Source: CAD feature listing. Evaluate the final solid. Frame: model axes, mm. A direction names the side the tool comes from. Give positions to 0.01 mm unless a question says otherwise; leave off trailing zeros. Order: outer loops, then holes, each group sorted by start corner. A loop starts at its lowest first (then second) coordinate and runs counter-clockwise, first axis right, second up.
```python
from build123d import *

# Parameters (mm, degrees)
SKETCH001_W   = 180
SKETCH001_H   = 136
SKETCH001_W_2 = 164.9
SKETCH001_H_2 = 124.27
PAD001_DEPTH  = 10
SKETCH_W      = 170
SKETCH_H      = 127
SKETCH_W_2    = 165
SKETCH_H_2    = 100
PAD_DEPTH     = 10
SKETCH002_R   = 1.5
POCKET_DEPTH  = 7
CHAMFER_SIZE  = 1


with BuildPart() as body001:
    # Sketch001 → Pad001 (new body)
    with BuildSketch(Plane.XY):
        Rectangle(SKETCH001_W, SKETCH001_H)
        Rectangle(SKETCH001_W_2, SKETCH001_H_2, mode=Mode.SUBTRACT)
    extrude(amount=PAD001_DEPTH)


with BuildPart() as body001_1:
    # Body001 placement: moved
    add(body001.part.moved(Location((0, 0, 2))))


with BuildPart() as bezel:
    # Sketch → Pad (new body)
    with BuildSketch(Plane.XY):
        Rectangle(SKETCH_W, SKETCH_H)
        Rectangle(SKETCH_W_2, SKETCH_H_2, mode=Mode.SUBTRACT)
    extrude(amount=PAD_DEPTH)

    # Boolean: cut Body001
    add(body001_1.part, mode=Mode.SUBTRACT)

    # Sketch002 (on Face18 of Boolean) → Pocket (cut)
    with BuildSketch(Plane.XY.offset(10)):
        with Locations((-78.09, 56.795)):
            Circle(SKETCH002_R)
        with Locations((78.09, 56.795)):
            Circle(SKETCH002_R)
        with Locations((78.09, -56.795)):
            Circle(SKETCH002_R)
        with Locations((-78.09, -56.795)):
            Circle(SKETCH002_R)
    extrude(amount=-POCKET_DEPTH, mode=Mode.SUBTRACT)

    # Chamfer
    chamfer_edges = [bezel.edges().sort_by_distance(p)[0] for p in [
        (82.5, 0, 0),
        (0, -50, 0),
        (0, -63.5, 0),
        (85, 0, 0),
        (0, 63.5, 0),
        (-85, 0, 0),
        (0, 50, 0),
        (-82.5, 0, 0),
    ]]
    chamfer(chamfer_edges, length=CHAMFER_SIZE)


solid = bezel.part
```
1) Section query C-C, the plane x = -18. Return the cut outline in (y, z) (3 decimals).
Report:
outline: (-63.5, 1) - (-62.5, 0) - (-51, 0) - (-50, 1) - (-50, 10) - (-62.135, 10) - (-62.135, 2) - (-63.5, 2) - close; (50, 1) - (51, 0) - (62.5, 0) - (63.5, 1) - (63.5, 2) - (62.135, 2) - (62.135, 10) - (50, 10) - close
2) Draft query along Y for faces 5 (the flat face through (-1, 62.135, 6)), 6 (the flat face through (-82.45, 56, 6)), 7 (the flat face through (-1, -50, 5)). Return one class per face: +Y half, -Y half, draft (parallel to the pull), parting line (faces both ways), or undercut.
Report:
face 5: +Y half
face 6: draft
face 7: undercut
3) Section query B-B, the plane z = 8.25. Return the cut outline in (x, y) (3 decimals), and give its area (3 significant figures).
Report:
outline: (-82.45, -62.135) - (82.45, -62.135) - (82.45, -50) - (-82.45, -50) - close; (-82.45, 50) - (82.45, 50) - (82.45, 62.135) - (-82.45, 62.135) - close; hole circle Ø3 at (-78.09, -56.795); hole circle Ø3 at (-78.09, 56.795); hole circle Ø3 at (78.09, -56.795); hole circle Ø3 at (78.09, 56.795)
area: 3,970 mm2
4) Material intervals for L1, parallel to Y at x = 78.09, z = 4.75 (3 decimals); L2, parallel to Y at x = 63, z = 5.5 (3 decimals); L3, parallel to X at y = 53.5, z = 6.5, sorted ascending.
Report:
L1: y = -62.135 to -58.295, -55.295 to -50, 50 to 55.295, 58.295 to 62.135
L2: y = -62.135 to -50, 50 to 62.135
L3: x = -82.45 to 82.45
5) Reachability of faces 1 (the flat face through (82.45, 56, 6)), 2 (the flat face through (-82.45, -56, 6)), 3 (the flat face through (-1, -62.135, 6)), 4 (the flat face through (-1, -56, 10)) from +Z, -Z, +X, -X, +Y, -Y: full face, straight path, thin tool, end or side. Return the list, or none.
Report:
face 1: +Z, +X, +Y, -Y
face 2: +Z, -X, +Y, -Y
face 3: +Z, +X, -X, -Y
face 4: +Z, +X, -X, +Y, -Y
6) Pin query (flat end, axial travel): pin 1 (1.5 mm diameter, centred on x = 28, z = 5, fed in from +Y) (3 decimals); pin 2 (0.9 mm diameter, centred on x = -78.5, y = -57, fed in from +Z); pin 3 (2.5 mm diameter, centred on y = 56.5, z = 6, fed in from +X). Return the tip coordinate at first contact, or that it passes through.
Report:
pin 1: stops at y = 62.135
pin 2: stops at z = 3
pin 3: stops at x = 82.45
7) Section query A-A, the plane y = 8. Return the cut outline in (x, z).
Report:
outline: (-85, 1) - (-84, 0) - (-83.5, 0) - (-82.5, 1) - (-82.5, 2) - (-85, 2) - close; (82.5, 1) - (83.5, 0) - (84, 0) - (85, 1) - (85, 2) - (82.5, 2) - close
